Autodesk Fusion 360 part; units mm, degrees
sketch "Sketch1" plane through (0, 0, 0) normal (1, 0, 0) x (0, 1, 0)
  line L0 (-5, 6) -> (11.1286, 6)
  line L1 (11.1286, 6) -> (11.1286, -7.5034)
  line L2 (11.1286, -7.5034) -> (-5, -7.5034)
  line L3 (-5, -7.5034) -> (-5, 6)
sketch "Sketch2" plane through (0, 0, 0) normal (1, 0, 0) x (0, 1, 0)
  line L0 (-28, 22) -> (-16, 22)
  line L1 (-16, 22) -> (-16, 10.6443)
  line L2 (-16, 10.6443) -> (-36, 10.6443)
  line L3 (-36, 10.6443) -> (-28, 22)
sketch "Sketch3" plane through (0, 0, 0) normal (0, 0, 1) x (1, 0, 0)
  circle A0 centre (-31.5, 17.5) radius 1.5811
sketch "Sketch4" plane through (0, 0, 0) normal (0, 0, 1) x (1, 0, 0)
  line L0 (-20, 25) -> (-5, 25)
  line L1 (-5, 25) -> (-5, 5)
  line L2 (-5, 5) -> (-20, 5)
  line L3 (-20, 5) -> (-20, 25)
sketch "Sketch5" plane through (0, 0, 2.8539) normal (0, 0, 1) x (-1, 0, 0)
  line L0 (20, -5) -> (5, -5)
  line L1 (5, -5) -> (5, -25)
  line L2 (5, -25) -> (20, -25)
  line L3 (20, -25) -> (20, -5)
  line L4 (13.5, -20) -> (10.5, -20)
  arc A0 (10.5, -18.5) -> (10.5, -20) centre (10.5, -19.25) ccw
  line L5 (10.5, -18.5) -> (13.5, -18.5)
  arc A1 (13.5, -20) -> (13.5, -18.5) centre (13.5, -19.25) ccw
sketch "Sketch6" plane through (0, 0, 2.8539) normal (0, 0, 1) x (-1, 0, 0)
  line L0 (13.5, -20) -> (10.5, -20)
  arc A0 (10.5, -18.5) -> (10.5, -20) centre (10.5, -19.25) ccw
  line L1 (10.5, -18.5) -> (13.5, -18.5)
  arc A1 (13.5, -20) -> (13.5, -18.5) centre (13.5, -19.25) ccw
  line L2 (20, -5) -> (5, -5)
  line L3 (5, -5) -> (5, -25)
  line L4 (5, -25) -> (20, -25)
  line L5 (20, -25) -> (20, -5)
  circle A2 centre (12, -7) radius 1
  dimension "d11" = 2
sketch "Sketch7" plane through (0, 0, 0) normal (0, 0, 1) x (1, 0, 0)
  line L0 (-5, 10) -> (-15, 10)
  line L1 (-15, 10) -> (-15, -32)
  line L2 (-15, -32) -> (-5, -32)
  line L3 (-5, -32) -> (-5, 10)
  dimension "d14" = 42
  dimension "d15" = 10
extrude "Extrude7" add sketch "Sketch7" along normal blind 2
sketch "Sketch8" plane through (0, 0, 2) normal (0, 0, 1) x (-1, 0, 0)
  line L0 (5, 32) -> (5, -10)
  line L1 (5, -10) -> (15, -10)
  line L2 (15, -10) -> (15, 32)
  line L3 (15, 32) -> (5, 32)
  circle A0 centre (10, -6.5) radius 1.5
  dimension "d18" = 3
extrude "Extrude8" cut sketch "Sketch8" against normal blind 7 contours A0
sketch "Sketch9" plane through (0, 0, 0) normal (0, 0, 1) x (1, 0, 0)
  line L0 (-15, -32) -> (-5, -32)
  line L1 (-15, 10) -> (-15, -32)
  line L2 (-12, -29) -> (-8, -29)
  line L3 (-8, -26) -> (-12, -26)
  ellipse E0 centre (-12, -27.5) end of major axis (-12, -29) minor radius 0.5003 (-12, -26) -> (-12, -29) ccw
  ellipse E1 centre (-8, -27.5) end of major axis (-8, -29) minor radius 0.5011 (-8, -29) -> (-8, -26) ccw
extrude "Extrude9" cut sketch "Sketch9" along normal blind 3.5
sketch "Sketch10" plane through (0, 0, 0) normal (0, 0, 1) x (1, 0, 0)
  line L0 (-5, 10) -> (-15, 10)
  line L1 (15, -15) -> (35, -15)
  line L2 (15, -15) -> (15, -5)
  line L3 (15, -5) -> (35, -5)
  line L4 (35, -5) -> (35, -15)
  dimension "d27" = 20
sketch "Sketch11" plane through (0, 0, 0) normal (1, 0, 0) x (0, 1, 0)
  line L0 (-32, 0) -> (10, 0)
  line L1 (-5, 0) -> (-5, 1)
  line L2 (-15, 0) -> (-5, 0)
  line L3 (-5, 0) -> (-7.5, 3)
  line L4 (-7.5, 3) -> (-12.5, 3)
  line L5 (-12.5, 3) -> (-15, 0)
  point P0 (-15, 0)
  point P1 (-15, 0)
sketch "Sketch12" plane through (0, 0, 0) normal (1, 0, 0) x (0, 1, 0)
  circle A0 centre (-2.5, 7.5) radius 1.25
  dimension "d32" = 2.5
sketch "Sketch13" plane through (16, 0, 0) normal (1, 0, 0) x (0, 1, 0)
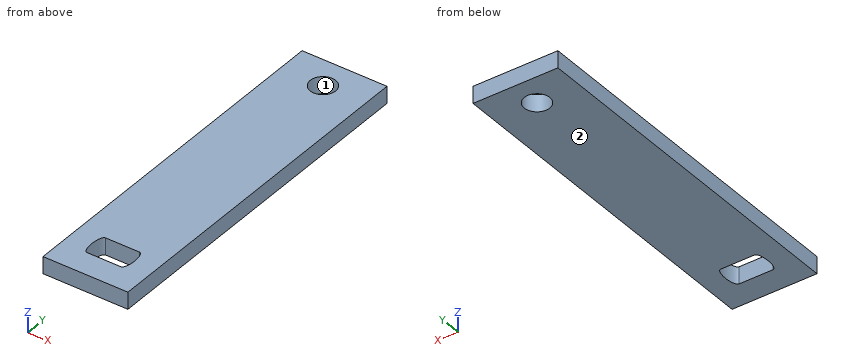
The listing builds one solid part. Answer for the finished solid, in the listing's coordinates (mm). Face numbers are marked on the shaded views. Coordinates: 2 decimals unless noted, no trailing zeros. Loops run counter-clockwise (first coordinate to the right, second up) from the corner with the lowest first, then second, coordinate; pieces in that order, holes last. Notation, with made-up numbers: (58, 42.5) -> (92, 42.5) arc R36 cw to (92, 76.5) -> close; hole circle Ø10 at (51.25, 39). An arc over 180 degrees is marked (long way). Use one line per item in the form item = value. Start each with the question number.
Item 1: The part is cut by section B-B on y = 6.5. Determine the outline of the cut face in (x, z), then the cut area to 3 significant figures.
Item 2: The part is cut by section C-C on z = 0.5. Count the separate pieces of the cut face and the enclosed holes in it, then the cut area to 3 significant figures.
Item 3: Consider L1, parallel to Y at x = -10, z = 0.5; L2, parallel to X at y = 6.5, z = 0.75; L3, parallel to Y at x = -8, z = 0.35. Determine where each line is inside the solid, lowest interval first. Write a range as [from, to].
Item 4: The mould has two halves that part along X. Classify the marked faces 1 and 2: released by +X, released by -X, zero draft, split by the parting line, or undercut.
Item 5: The part is cut by section A-A on x = -10. Determine the outline of the cut face in (y, z), then the cut area to 3 significant figures.
Answer key:
q1.outline = (-15, 0) -> (-11.5, 0) -> (-11.5, 2) -> (-15, 2) -> close; (-8.5, 0) -> (-5, 0) -> (-5, 2) -> (-8.5, 2) -> close
q1.area = 14.0 mm2
q2.separate_pieces = 1
q2.enclosed_holes = 2
q2.area = 399 mm2
q3.L1 = [-32, -29], [-26, 5], [8, 10]
q3.L2 = [-15, -11.5], [-8.5, -5]
q3.L3 = [-32, -29], [-26, 10]
q4.face_1 = undercut
q4.face_2 = zero draft
q5.outline = (-32, 0) -> (-29, 0) -> (-29, 2) -> (-32, 2) -> close; (-26, 0) -> (5, 0) -> (5, 2) -> (-26, 2) -> close; (8, 0) -> (10, 0) -> (10, 2) -> (8, 2) -> close
q5.area = 72.0 mm2
